Could you check a few things on this model? Use its own coordinates, in mm. Coordinates: 2 decimals unless noted, no trailing zeros. Loops run counter-clockwise (first coordinate to the right, second up) from the corner with the lowest first, then second, coordinate; pieces in that order, holes last. Notation, with made-up numbers: (54.5, -1) -> (59.5, -1) arc R12 ccw to (59.5, 3) -> close; hole circle Ø1 at (12.25, -1). An arc over 180 degrees is marked (long way). One line per question, with ' | ' between items. Start each with the question number.
(1) If I drill on line 1 along Z through (x, y) = (166, 7.5); line 2 along X through (y, z) = (3.25, 388.5); line 3 along X through (y, z) = (23.5, 396), over which ranges is the centre line in solid material (lowest first)?
(2) I'm going to push flat-ended pins straight in: pin 1 Ø13 at (x, y) = (-28, 9) entering from +Z; pin 2 Ø1.5 at (y, z) = (16, 332) entering from +X; pin 3 Ø12 at (y, z) = (18.5, 331.5) entering from -X. Where does each tip first touch, or does it pass through?
(3) Suppose I cut it at B-B (y = 16.5). Please give me the cut outline in (x, z), plus the area to 3 significant figures.
(4) Suppose I cut it at A-A (z = 386). Please give me the cut outline in (x, y).
(5) Suppose I cut it at D-D (z = 328.5). Please give me the cut outline in (x, y).
(6) Suppose I cut it at C-C (x = -134). Please give me the cut outline in (y, z).
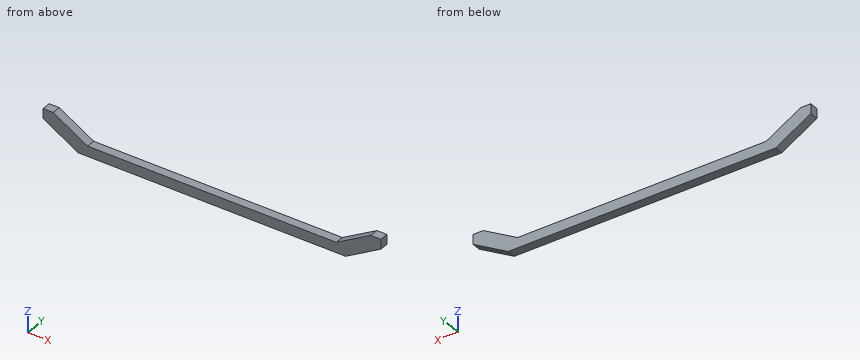
Autodesk Inventor part; units mm, degrees
ref_plane "YZ Plane" through (0, 0, 0) normal (1, 0, 0) x (0, 1, 0)
ref_plane "XZ Plane" through (0, 0, 0) normal (0, 1, 0) x (-1, 0, 0)
ref_plane "XY Plane" through (0, 0, 0) normal (0, 0, 1) x (1, 0, 0)
sketch "Sketch1" plane through (0, 0, 0) normal (0, 1, 0) x (-1, 0, 0)
  line L0 (555.2926, 403.499) -> (-444.7074, 403.499)
  line L1 (-444.7074, 403.499) -> (-444.7074, 314.499)
  line L2 (-444.7074, 314.499) -> (555.2926, 314.499)
  line L3 (555.2926, 314.499) -> (555.2926, 403.499)
  line L4 (423.1016, 344.499) -> (-312.5164, 344.499)
  line L5 (-444.7074, 403.499) -> (-414.7074, 403.499)
  line L6 (-414.7074, 403.499) -> (-414.7074, 374.7123)
  line L7 (-414.7074, 374.7123) -> (-444.7074, 374.7123)
  line L8 (-444.7074, 374.7123) -> (-444.7074, 403.499)
  line L9 (555.2926, 403.499) -> (525.2926, 403.499)
  line L10 (525.2926, 403.499) -> (525.2926, 374.7123)
  line L11 (525.2926, 374.7123) -> (555.2926, 374.7123)
  line L12 (555.2926, 374.7123) -> (555.2926, 403.499)
  line L13 (525.2926, 403.499) -> (423.1016, 344.499)
  line L14 (-414.7074, 403.499) -> (-312.5164, 344.499)
  line L15 (-444.7074, 374.7123) -> (-340.4148, 314.499)
  line L16 (555.2926, 374.7123) -> (451, 314.499)
  point P0 (0, 0)
  point P1 (555.2926, 368.7138)
  point P2 (522.9975, 314.499)
  point P3 (-444.7074, 354.0015)
  point P4 (-397.9975, 314.499)
  point P5 (525.2926, 403.499)
  point P6 (525.2926, 403.499)
  dimension "d0" = 1000
  dimension "d5" = 30
  dimension "d11" = 89
  dimension "d12" = 30
  dimension "d13" = 30
  dimension "d17" = 60
  dimension "d18" = 60
extrude "Extrusion1" add sketch "Sketch1" along normal blind 26 contours L3 L11 L10 L0 | L10 L11 L16 L2 L15 L7 L6 L14 L4 L13 | L6 L7 L1 L0
sketch "Sketch2" plane through (0, 26, 0) normal (0, 1, 0) x (1, 0, 0)
  point P0 (0, 0)
properties part number "UcreplenieX" material "Aluminum 6061"
Checks:
1) line 1: z = 314.5 to 344.5 | line 2: x = -555.29 to -499.31, 388.73 to 444.71 | line 3: x = -555.29 to -512.3, 401.72 to 444.71
2) pin 1: stops at z = 344.5 | pin 2: stops at x = 372.03 | pin 3: stops at x = -490.84
3) outline: (-555.29, 374.71) -> (-451, 314.5) -> (340.41, 314.5) -> (444.71, 374.71) -> (444.71, 403.5) -> (414.71, 403.5) -> (312.52, 344.5) -> (-423.1, 344.5) -> (-525.29, 403.5) -> (-555.29, 403.5) -> close | area: 33,300 mm^2
4) outline: (-555.29, 0) -> (-494.98, 0) -> (-494.98, 26) -> (-555.29, 26) -> close; (384.4, 0) -> (444.71, 0) -> (444.71, 26) -> (384.4, 26) -> close
5) outline: (-475.25, 0) -> (364.67, 0) -> (364.67, 26) -> (-475.25, 26) -> close
6) outline: (0, 314.5) -> (26, 314.5) -> (26, 344.5) -> (0, 344.5) -> close
